Build history of the part. All positions in model axes, mm. A direction names the side the tool comes from. Round coordinates to 2 decimals unless told otherwise and drop trailing zeros. Loops run counter-clockwise (first coordinate to the right, second up) from the corner with the lowest first, then second, coordinate; pieces in that order, holes last. Notation, with made-up numbers: (-35, 16.25) - (-15, 16.25) arc R15 cw to (-15, 24.25) - close; hole circle Ø3 at (-6.5, 38.25). An arc over 180 degrees is marked (long way). Answer as CSV lines item,"result". Start each with the question number.
Autodesk Inventor part; units mm, degrees
ref_plane "YZ Plane" through (0, 0, 0) normal (1, 0, 0) x (0, 1, 0)
ref_plane "XZ Plane" through (0, 0, 0) normal (0, 1, 0) x (-1, 0, 0)
ref_plane "XY Plane" through (0, 0, 0) normal (0, 0, 1) x (1, 0, 0)
sketch "Sketch1" plane through (0, 0, 0) normal (0, 0, 1) x (1, 0, 0)
  line L0 (-8, -2) -> (-2, -2)
  line L1 (-2, -2) -> (-8, -2)
  line L2 (-2, -2) -> (-2, -7.923)
  line L3 (2, -8) -> (2, -2.0038)
  line L4 (2, -2.0038) -> (2, -8)
  arc A0 (8, -2.0038) -> (10.0019, 0) centre (8, -0.0019) ccw
  line L5 (2, -2.0038) -> (8, -2.0038)
  line L6 (2, 2) -> (2, 8)
  line L7 (8, 2) -> (2, 2)
  line L8 (2, 2) -> (8, 2)
  line L9 (2, 2) -> (2, 8)
  line L10 (-2, 8) -> (-2, 2)
  line L11 (-2, 2) -> (-2, 8)
  arc A1 (-8, 2) -> (-10, 0) centre (-8, 0) ccw
  line L12 (-2, 2) -> (-8, 2)
  arc A2 (-8, 2) -> (-8, -2) centre (-8, 0) ccw
  arc A3 (-2, -8) -> (0, -10) centre (0, -8) ccw
  arc A4 (-2, -8) -> (2, -8) centre (0, -8) ccw
  arc A5 (8, -2.0038) -> (8, 2) centre (8, -0.0019) ccw
  arc A6 (2, 8) -> (-2, 8) centre (0, 8) ccw
  circle A7 centre (0, 0) radius 11.5
  line L13 (-2, 2) -> (-2.3536, 2.3536)
  line L14 (-2, 2) -> (-1.5, 2) construction
  line L15 (-2.3536, 2.3536) -> (-8, 2.3536)
  line L16 (-8, 2.3536) -> (-8, 2)
  line L17 (-2, -2) -> (-2.3536, -2.3536)
  line L18 (-2.3536, -2.3536) -> (-8, -2.3536)
  line L19 (-8, -2.3536) -> (-8, -2)
  line L20 (-2.3536, -2.3536) -> (-2.3536, -8)
  line L21 (-2.3536, -8) -> (-2, -8)
  line L22 (2, -2.0038) -> (2.3536, -2.3573)
  line L23 (2.3536, -2.3573) -> (2.3536, -8)
  line L24 (2.3536, -8) -> (2, -8)
  line L25 (-2, -7.923) -> (-2, -8)
  line L26 (2.3536, -2.3573) -> (8, -2.3573)
  line L27 (8, -2.3573) -> (8, -2.0038)
  line L28 (2, 2) -> (2.3536, 2.3536)
  line L29 (2.3536, 2.3536) -> (8, 2.3536)
  line L30 (8, 2.3536) -> (8, 2)
  line L31 (2.3536, 2.3536) -> (2.3536, 8)
  line L32 (2.3536, 8) -> (2, 8)
  line L33 (-2.3536, 2.3536) -> (-2.3536, 8)
  line L34 (-2.3536, 8) -> (-2, 8)
  arc A8 (2.3536, 8) -> (-2.3536, 8) centre (0, 8) ccw
  arc A9 (8, -2.3573) -> (8, 2.3536) centre (8, -0.0019) ccw
  arc A10 (-2.3536, -8) -> (2.3536, -8) centre (0, -8) ccw
  arc A11 (-8, 2.3536) -> (-8, -2.3536) centre (-8, 0) ccw
  line L35 (-2, 2) -> (-2.0707, 2.0707)
  line L36 (-2.0707, 2.0707) -> (-8, 2.0707)
  line L37 (-2.0707, 2.0707) -> (-2.0707, 8)
  line L38 (-2, -2) -> (-2.0707, -2.0707)
  line L39 (-2.0707, -2.0707) -> (-8, -2.0707)
  line L40 (-2.0707, -2.0707) -> (-2.0354, -8)
  line L41 (2, -2.0038) -> (2.0707, -2.0745)
  line L42 (2.0707, -2.0745) -> (2.0707, -8)
  line L43 (2.0707, -2.0745) -> (8, -2.0745)
  line L44 (2, 2) -> (2.0707, 2.0707)
  line L45 (2.0707, 2.0707) -> (8, 2.0707)
  line L46 (2.0707, 2.0707) -> (2.0707, 8)
  arc A12 (2.0707, 8) -> (-2.0707, 8) centre (0, 8) ccw
  arc A13 (-8, 2.0707) -> (-8, -2.0707) centre (-8, 0) ccw
  arc A14 (-2.0354, -8) -> (2.0707, -8) centre (0.0177, -8) ccw
  arc A15 (8, -2.0745) -> (8, 2.0707) centre (8, -0.0019) ccw
  line L47 (-11.5, 11.5) -> (11.5, 11.5)
  line L48 (11.5, 11.5) -> (11.5, -11.5)
  line L49 (11.5, -11.5) -> (-11.5, -11.5)
  line L50 (-11.5, -11.5) -> (-11.5, 11.5)
  point P0 (-11.5, 0)
  point P1 (0, -11.5)
  point P2 (0, 11.5)
  point P3 (11.5, 0)
  dimension "d1" = 23
  dimension "d2" = 0.5
  dimension "d3" = 135
  dimension "d4" = 0.5
  dimension "d6" = 5.6464
  dimension "d7" = 5.6464
  dimension "d8" = 0.5
  dimension "d9" = 0.5
  dimension "d10" = 0.1
  dimension "d11" = 0.1
  dimension "d13" = 0.1
  dimension "d14" = 0.1
  dimension "d22" = 23
  dimension "d23" = 23
extrude "Extrusion1" add sketch "Sketch1" along normal blind 10 contours L39 L17 L18 L19 | L19 A11 L16 A13 | L40 L21 L20 L17 | L16 L15 L13 L36 | A14 L24 A10 L21 | L13 L33 L34 L37 | L42 L22 L23 L24 | L34 A8 L32 A12 | L43 L27 L26 L22 | L32 L31 L28 L46 | A15 L30 A9 L27 | L28 L29 L30 L45 | A7 | L48 L49 A7 | A7 L47 L48 | A7 L50 L47 | L49 L50 A7
extrude "Extrusion2" add sketch "Sketch1" against normal blind 150 contours A2 A1 L12 L10 A6 L6 L7 A5 A0 L5 L3 A4 A3 L25 L2 L0 | L19 A13 L16 A1 A2 | L0 L17 L39 L19 | L2 L25 L21 L40 L17 | L39 L17 L18 L19 | L19 A11 L16 A13 | L40 L21 L20 L17 | L16 L36 L13 L12 | L16 L15 L13 L36 | A3 A4 L24 A14 L21 | A14 L24 A10 L21 | L13 L37 L34 L10 | L13 L33 L34 L37 | L42 L22 L23 L24 | L24 L3 L22 L42 | L34 A12 L32 A6 | L34 A8 L32 A12 | L43 L27 L26 L22 | L22 L5 L27 L43 | L32 L46 L28 L6 | L32 L31 L28 L46 | A15 L30 A9 L27 | L27 A0 A5 L30 A15 | L28 L45 L30 L7 | L28 L29 L30 L45 | A7 | L48 L49 A7 | A7 L47 L48 | A7 L50 L47 | L49 L50 A7
sketch "Sketch2" plane through (0, 0, -150) normal (0, 0, -1) x (-1, 0, 0)
  circle A0 centre (0, 0) radius 2.3
  dimension "d19" = 4.6
extrude "Extrusion3" cut sketch "Sketch2" against normal blind 6
properties part number "Tussen stuk V1.1" material "ABS Plastic"
Q1. Band-saw the part on A-A, the plane y = 0. List the corners of the cut face in (x, z).
Q2. Wall check: probe 1 along Y at (x, z) = (0, -145.3); probe 2 along Y at (x, z) = (6.5, 0.5); probe 3 along Z at (x, y) = (0.5, 2.5). Give the ranges that are in metal, low to high. Write a range as [from, to].
Q3. Tool access for faces 1 (the cylindrical face through (10.072, 0.044, 4.93)), 2 (the cylindrical face through (1.825, -1.4, -147.042)), 3 (the flat face through (0, 11.5, -71)): list every direction of +Z, -Z, +X, -X, +Y, -Y with a clear straight run to the whole face (end or side of a thin tool).
Q4. Two-plate mould, pull along Y, no slides. Class faces 4 (the flat face through (5, 2.071, 5)), 5 (the flat face through (0, -11.5, -71)), 6 (the flat face through (-11.5, 0, -71)): released by +Y, released by -Y, zero draft, split by the parting line, or undercut.
Q5. Pin check, flat tip, straight feed: pin 1 Ø2.5 at (x, y) = (0, -1) entering from -Z. Stop position of the tip, or through.
Q6. Band-saw the part on B-B, the plane x = 0. List the corners of the cut face in (y, z), then the cut area to 3 significant figures.
Reported:
1,outline,"(-11.5, -150) - (-2.3, -150) - (-2.3, -144) - (2.3, -144) - (2.3, -150) - (11.5, -150) - (11.5, 10) - (10.07, 10) - (10.07, 0) - (-10.07, 0) - (-10.07, 10) - (-11.5, 10) - close"
2,probe 1,"y = [-11.5, -2.3], [2.3, 11.5]"
2,probe 2,"y = [-11.5, -2.07], [2.07, 11.5]"
2,probe 3,"z = [-150, 0]"
3,face 1,"+Z"
3,face 2,"-Z"
3,face 3,"+Z, -Z, +X, -X, +Y"
4,face 4,"undercut"
4,face 5,"released by -Y"
4,face 6,"zero draft"
5,pin 1,"stops at z = -144"
6,outline,"(-11.5, -150) - (-2.3, -150) - (-2.3, -144) - (2.3, -144) - (2.3, -150) - (11.5, -150) - (11.5, 10) - (10.07, 10) - (10.07, 0) - (-10.05, 0) - (-10.05, 10) - (-11.5, 10) - close"
6,area,"3,450 mm2"
